Verification items for the finished model (mm, model axes). Face numbers are marked on the shaded views. A direction names the side the tool comes from. Coordinates: 2 decimals unless noted, no trailing zeros. Order: outer loops, then holes, each group sorted by start corner. A loop starts at its lowest first (then second) coordinate and runs counter-clockwise, first axis right, second up. Notation, with made-up numbers: M 47.25,75 L 62.25,75 A36 cw 62.25,111 Z; hole C -19.75,45 d6. An arc over 180 degrees is marked long. Return JSON: item names as keys, results as strings. Group by question number.
1. Mould release check, pull along Y, two halves, no side actions. Record for the marked faces 1, 2 and 3: +Y half, -Y half, draft (parallel to the pull), parting line (faces both ways), or undercut.
2. Section check A-A, the plane z = 8.5. Record the cut outline in (x, y), plus the area to 3 significant figures.
3. Gauge pin test, flat ends, axial feed: pin 1 (20 mm diameter, centred on x = 442.5, y = 37.5, fed in from -Z); pin 2 (2 mm diameter, centred on x = 452.5, z = 9.5, fed in from -Y); pin 3 (2 mm diameter, centred on x = 447, y = 30, fed in from +Z). Record the tip position at first contact, or that the pin passes through.
4. Material ranges on line 1 along Y through (x, z) = (451.25, 7); line 2 along Z through (x, y) = (443.25, 0); line 3 along Z through (x, y) = (450, 0), recorded low to high.
5. Set-up check for the marked faces 4, 5, 6, 7 and 8: record each of +Z, -Z, +X, -X, +Y, -Y from which the full face is reachable in a straight line by a thin tool's end or side.
6. Section check B-B, the plane z = -13.5. Record the cut outline in (x, y), plus the area to 3 significant figures.
7. Section check C-C, the plane y = 41. Record the cut outline in (x, z).
```python
from build123d import *

# Parameters (mm, degrees)
AUFSATZ_LINEAR_START             = -2.5
SKIZZE2_R                        = 25
AUFSATZ_LINEAR_AUSTRAGEN1_DEPTH  = 6
AUFSATZ_LINEAR_START_2           = -5.5
AUFSATZ_LINEAR_AUSTRAGEN6_DEPTH  = 3
SCHNITT_LINEAR_AUSTRAGEN2_DEPTH  = 478.699958133
AUFSATZ_LINEAR_START_3           = -2.916019
AUFSATZ_LINEAR_AUSTRAGEN5_DEPTH  = 16.916019
SPIEGELN4_START                  = -2.916018908
SPIEGELN4_DEPTH                  = 16.916018908
F_6_4_6_4_DURCHMESSER_BOHRUNG1_D = 6.4
VERRUNDUNG2_R                    = 1


# Read off the part's stored shape, not the designer's step: Spiegeln4
with BuildPart() as part:
    # Skizze2 → Aufsatz-Linear austragen1 (new body)
    with BuildSketch(Plane.XY.offset(AUFSATZ_LINEAR_START)):
        with Locations((450, 0)):
            Circle(SKIZZE2_R)
    extrude(amount=-AUFSATZ_LINEAR_AUSTRAGEN1_DEPTH)

    # Skizze10 → Aufsatz-Linear austragen6 (add)
    with BuildSketch(Plane.XY.offset(AUFSATZ_LINEAR_START_2)):
        with BuildLine():
            Line((448.038494427, 24.922931126), (445.796483155, 34.115177342))
            ThreePointArc((445.796483155, 34.115177342), (437.867394378, 49.743683049), (438.024320445, 32.2195279))
            Line((438.024320445, 32.2195279), (440.266331717, 23.027281684))
            ThreePointArc((440.266331717, 23.027281684), (444.076095495, 24.28800847), (448.038494427, 24.922931126))
        make_face()
    extrude(amount=AUFSATZ_LINEAR_AUSTRAGEN6_DEPTH)

    # Skizze8 → Schnitt-Linear austragen2 (cut, symmetric)
    with BuildSketch(Plane(origin=(0, 0, 0), x_dir=(1, 0, 0), z_dir=(0, 1, 0))):
        with BuildLine():
            Line((475, 2.5), (450, 2.5))
            ThreePointArc((450, 2.5), (462.527846235, 2.917876468), (475, 4.169648205))
            Line((475, 4.169648205), (475, 2.5))
        make_face()
    schnitt_linear_austragen2 = extrude(amount=SCHNITT_LINEAR_AUSTRAGEN2_DEPTH, both=True, mode=Mode.SUBTRACT)

    # Spiegeln1: Schnitt-Linear austragen2 across plane
    add(schnitt_linear_austragen2.mirror(Plane(origin=(450, 0, 0), x_dir=(0, 0, 1), z_dir=(1, 0, 0))), mode=Mode.SUBTRACT)

    # Skizze3 → Aufsatz-Linear austragen5 (add)
    with BuildSketch(Plane.XY.offset(AUFSATZ_LINEAR_START_3)):
        with BuildLine():
            Line((450, 0), (462.5, 0))
            ThreePointArc((462.5, 0), (460.303300859, 5.303300859), (455, 7.5))
            Line((455, 7.5), (450, 7.5))
            Line((450, 7.5), (450, 0))
        make_face()
    extrude(amount=AUFSATZ_LINEAR_AUSTRAGEN5_DEPTH)

    # Spiegeln4 outline → Spiegeln4 (add)
    with BuildSketch(Plane.XY.offset(SPIEGELN4_START)):
        with BuildLine():
            ThreePointArc((455, -7.5), (460.303300859, -5.303300859), (462.5, 0))
            Line((462.5, 0), (450, 0))
            Line((450, 0), (450, 7.5))
            Line((450, 7.5), (445, 7.5))
            ThreePointArc((445, 7.5), (437.5, 0), (445, -7.5))
            Line((445, -7.5), (455, -7.5))
        make_face()
    extrude(amount=SPIEGELN4_DEPTH)

    # Skizze4 → Rotation1 (revolve)
    with BuildSketch(Plane(origin=(450, 0, 0), x_dir=(0, 0, -1), z_dir=(1, 0, 0)), mode=Mode.PRIVATE) as rotation1_sk:
        Polygon((9.5, 7), (8.5, 7), (8.5, 0), (18.5, 0), (18.5, 4), (18.5, 5), (9.5, 5), align=None)
    revolve(rotation1_sk.sketch.rotate(Axis((450, 0, -8.5), (0, 0, -1)), 90), axis=Axis((450, 0, -8.5), (0, 0, -1)))

    # Ø6.4 (6.4) Durchmesser Bohrung1 (through all)
    with Locations(Plane(origin=(462.5, 0, 0), x_dir=(0, 0, -1), z_dir=(1, 0, 0))):
        with Locations((-7, 0)):
            Hole(F_6_4_6_4_DURCHMESSER_BOHRUNG1_D / 2)

    # Verrundung2
    verrundung2_edges = [part.edges().sort_by_distance(p)[0] for p in [
        (437.5, 0, 14),
        (445, 0, -18.5),
        (425, 0, -8.5),
        (460.303300859, 5.303300859, 14),
        (450, 7.5, 14),
        (450, -7.5, 14),
    ]]
    fillet(verrundung2_edges, radius=VERRUNDUNG2_R)


solid = part.part
```
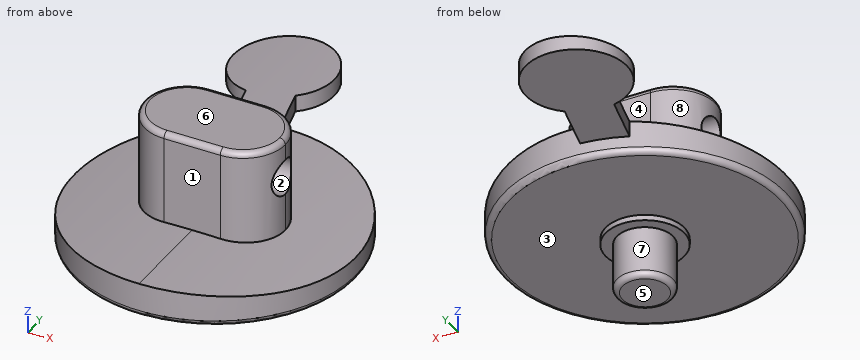
Answers follow:
{
 "1": {"face 1": "-Y half", "face 2": "undercut", "face 3": "draft"},
 "2": {"outline": "M 438.05,-2.83 A7.5 ccw 445,-7.5 L 455,-7.5 A7.5 ccw 461.95,-2.83 Z; M 438.05,2.83 L 461.95,2.83 A7.5 ccw 455,7.5 L 445,7.5 A7.5 ccw Z", "area": "187 mm^2"},
 "3": {"pin 1": "z = -5.5", "pin 2": "y = -7.5", "pin 3": "z = -2.52"},
 "4": {"line 1": "-7.5 to -3.2, 3.2 to 7.5", "line 2": "-9.5 to 3.8, 10.2 to 14", "line 3": "-18.5 to 3.8, 10.2 to 14"},
 "5": {"face 4": "+Z, +X, -X, +Y", "face 5": "-Z, +X, -X, +Y, -Y", "face 6": "+Z, +X, -X, +Y, -Y", "face 7": "-Z", "face 8": "+Z, -X"},
 "6": {"outline": "C 450,0 d10", "area": "78.5 mm^2"},
 "7": {"outline": "M 431,-5.5 L 449,-5.5 L 449,-2.5 A188 ccw 431,-3.46 Z"}
}
